Here's the drawing with two shaded views (mm, measured from the low corner). I have some questions. A direction names the side the tool comes from. Round coordinates to 2 decimals unless told otherwise and drop trailing zeros. Loops run counter-clockwise (first coordinate to the right, second up) from the corner with the lowest first, then second, coordinate; pieces in that order, holes last. Notation, with made-up numbers: (-1, 52) - (38, 52) arc R28 cw to (38, 78) - close; hole circle Ø10 at (-7, 13.5). An arc over 180 degrees is marked (long way). Use one line per item in the form item = value.
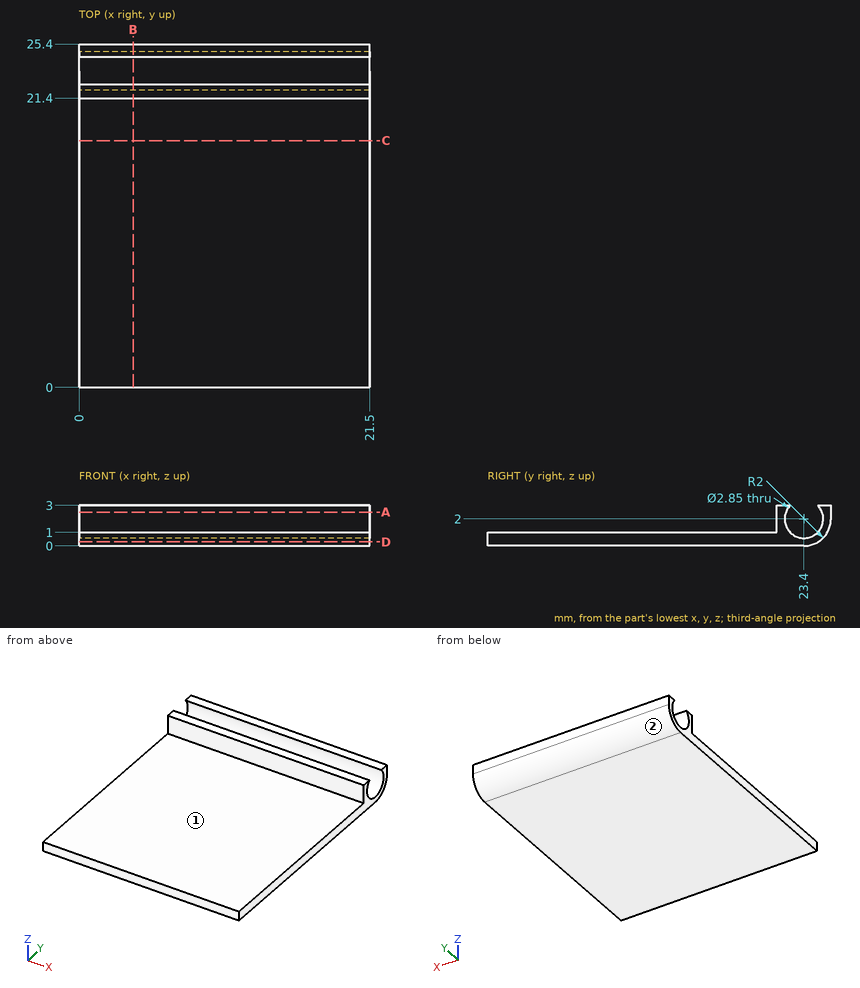
1. For P1, Ø10, axis at x = 11.5, y = 8, coming from the +Z side; P2, Ø1.6, axis at x = 10.5, z = 2.5, coming from the -Y side; P3, Ø1, axis at y = 5, z = 2, coming from the -X side, each with a flat end and sliding along its axis, tell me the tip position at first contact or that it passes through.
Solution:
P1 = 1
P2 = 21.4
P3 = through
2. If we section it at C-C, the plane y = 18.25: Write out the boundary of the cut face in (x, z), plus the area to 3 significant figures.
Solution:
outline = (0, 0) - (21.5, 0) - (21.5, 1) - (0, 1) - close
area = 21.5 mm^2
3. On a 3-axis mill with a long thin cutter (end or side, diameter ignored), from which of +Z, -Z, +X, -X, +Y, -Y can I reach the whole of each face in a straight line? I mean the marked faces 1 and 2. Say none if no direction works.
Solution:
face_1 = +Z, +X, -X, -Y
face_2 = -Z, +X, -X, +Y
4. If we section it at B-B, the plane x = 4: Write out the boundary of the cut face in (y, z) (3 decimals), plus the area to 3 significant figures.
Solution:
outline = (0, 0) - (23.4, 0) arc R2 ccw to (25.4, 2) - (25.4, 3) - (24.415, 3) arc R1.425 cw (long way) to (22.385, 3) - (21.4, 3) - (21.4, 1) - (0, 1) - close
area = 26.8 mm^2
5. If we section it at D-D, the plane z = 0.3: Write out the boundary of the cut face in (x, y), plus the area to 3 significant figures.
Solution:
outline = (0, 0) - (21.5, 0) - (21.5, 24.45) - (0, 24.45) - close
area = 526 mm^2
6. If we section it at A-A, the plane z = 2.5: Write out the boundary of the cut face in (x, y).
Solution:
outline = (0, 21.4) - (21.5, 21.4) - (21.5, 22.07) - (0, 22.07) - close; (0, 24.73) - (21.5, 24.73) - (21.5, 25.4) - (0, 25.4) - close
7. Please list where these lines run through material, in increasing order: line 1 along Y through (x, z) = (7.5, 2) (3 decimals); line 2 along Z through (x, y) = (13, 23.4) (3 decimals); line 3 along Z through (x, y) = (11.5, 5).
Solution:
line_1 = 21.4 to 21.975, 24.825 to 25.4
line_2 = 0 to 0.575
line_3 = 0 to 1
